from build123d import *

# Parameters (mm, degrees)
SKETCH1_R           = 16
SKETCH1_R_2         = 1.5
SKETCH1_R_3         = 5.25
SKETCH1_R_4         = 3
BOSS_EXTRUDE2_DEPTH = 3
SKETCH1_8_R         = 16
BOSS_EXTRUDE4_DEPTH = 10
SKETCH1_10_R        = 3
SKETCH1_10_R_2      = 1.5
BOSS_EXTRUDE6_DEPTH = 3
BOSS_EXTRUDE7_START = 3
SKETCH1_11_R        = 16
BOSS_EXTRUDE7_DEPTH = 57
CUT_EXTRUDE2_START  = -70
SKETCH2_R           = 1.5
CUT_EXTRUDE2_DEPTH  = 5


with BuildPart() as part:
    # Sketch1 → Boss-Extrude2 (new body)
    with BuildSketch(Plane(origin=(0, 0, 0), x_dir=(0, 0, -1), z_dir=(1, 0, 0))):
        Circle(SKETCH1_R)
        with Locations((0, 8.5)):
            Circle(SKETCH1_R_2, mode=Mode.SUBTRACT)
        with Locations((0, -8.5)):
            Circle(SKETCH1_R_2, mode=Mode.SUBTRACT)
        Circle(SKETCH1_R_3, mode=Mode.SUBTRACT)
        with Locations((8.5, 0)):
            Circle(SKETCH1_R_4, mode=Mode.SUBTRACT)
        with Locations((-8.5, 0)):
            Circle(SKETCH1_R_4, mode=Mode.SUBTRACT)
    extrude(amount=BOSS_EXTRUDE2_DEPTH)

    # Sketch1<8> → Boss-Extrude4 (add)
    with BuildSketch(Plane(origin=(0, 0, 0), x_dir=(0, 0, -1), z_dir=(1, 0, 0))):
        Circle(SKETCH1_8_R)
        with BuildLine():
            ThreePointArc((2.652911728, 9.900735294), (7.247844507, 7.247844507), (9.900735294, 2.652911728))
            ThreePointArc((9.900735294, 2.652911728), (11.069261166, 1.548837325), (11.5, 0))
            ThreePointArc((11.5, 0), (11.069261166, -1.548837325), (9.900735294, -2.652911728))
            ThreePointArc((9.900735294, -2.652911728), (7.247844507, -7.247844507), (2.652911728, -9.900735294))
            ThreePointArc((2.652911728, -9.900735294), (0, -11.5), (-2.652911728, -9.900735294))
            ThreePointArc((-2.652911728, -9.900735294), (-7.247844507, -7.247844507), (-9.900735294, -2.652911728))
            ThreePointArc((-9.900735294, -2.652911728), (-11.5, 0), (-9.900735294, 2.652911728))
            ThreePointArc((-9.900735294, 2.652911728), (-7.247844507, 7.247844507), (-2.652911728, 9.900735294))
            ThreePointArc((-2.652911728, 9.900735294), (0, 11.5), (2.652911728, 9.900735294))
        make_face(mode=Mode.SUBTRACT)
    extrude(amount=-BOSS_EXTRUDE4_DEPTH)

    # Sketch1<10> → Boss-Extrude6 (add)
    with BuildSketch(Plane(origin=(0, 0, 0), x_dir=(0, 0, -1), z_dir=(1, 0, 0))):
        with Locations((8.5, 0)):
            Circle(SKETCH1_10_R)
        with Locations((8.5, 0)):
            Circle(SKETCH1_10_R_2, mode=Mode.SUBTRACT)
        with Locations((-8.5, 0)):
            Circle(SKETCH1_10_R)
        with Locations((-8.5, 0)):
            Circle(SKETCH1_10_R_2, mode=Mode.SUBTRACT)
    extrude(amount=BOSS_EXTRUDE6_DEPTH)

    # Sketch1<11> → Boss-Extrude7 (add)
    with BuildSketch(Plane(origin=(0, 0, 0), x_dir=(0, 0, -1), z_dir=(1, 0, 0)).offset(BOSS_EXTRUDE7_START)):
        Circle(SKETCH1_11_R)
        with BuildLine():
            ThreePointArc((2.652911728, 9.900735294), (7.247844507, 7.247844507), (9.900735294, 2.652911728))
            ThreePointArc((9.900735294, 2.652911728), (11.069261166, 1.548837325), (11.5, 0))
            ThreePointArc((11.5, 0), (11.069261166, -1.548837325), (9.900735294, -2.652911728))
            ThreePointArc((9.900735294, -2.652911728), (7.247844507, -7.247844507), (2.652911728, -9.900735294))
            ThreePointArc((2.652911728, -9.900735294), (0, -11.5), (-2.652911728, -9.900735294))
            ThreePointArc((-2.652911728, -9.900735294), (-7.247844507, -7.247844507), (-9.900735294, -2.652911728))
            ThreePointArc((-9.900735294, -2.652911728), (-11.5, 0), (-9.900735294, 2.652911728))
            ThreePointArc((-9.900735294, 2.652911728), (-7.247844507, 7.247844507), (-2.652911728, 9.900735294))
            ThreePointArc((-2.652911728, 9.900735294), (0, 11.5), (2.652911728, 9.900735294))
        make_face(mode=Mode.SUBTRACT)
    extrude(amount=BOSS_EXTRUDE7_DEPTH)

    # Sketch2 → Cut-Extrude2 (cut)
    with BuildSketch(Plane.ZY.offset(10).offset(CUT_EXTRUDE2_START)):
        with Locations(Location((9.222798741, 9.222798741, 0), (0, 0, 180))):
            Circle(SKETCH2_R)
        with Locations(Location((-9.222798741, 9.222798741, 0), (0, 0, 180))):
            Circle(SKETCH2_R)
        with Locations(Location((9.222798741, -9.222798741, 0), (0, 0, 180))):
            Circle(SKETCH2_R)
        with Locations(Location((-9.222798741, -9.222798741, 0), (0, 0, 180))):
            Circle(SKETCH2_R)
    extrude(amount=CUT_EXTRUDE2_DEPTH, mode=Mode.SUBTRACT)


solid = part.part
Read the model definition and answer for the solid it produces. Units are mm, in the model's axes. A direction names the side the tool comes from. Coordinates: 2 decimals unless noted, no trailing zeros. Loops run counter-clockwise (first coordinate to the right, second up) from the corner with the lowest first, then second, coordinate; pieces in that order, holes last.
Q1. Consider probe 1 along Y at (x, z) = (42, 0); probe 2 along Y at (x, z) = (11, 1); probe 3 along Z at (x, y) = (50.5, -10). Determine where each line is inside the solid, lowest interval first.
Q2. The part is cut by section D-D on y = 8.5. Write down the section's boundary in (x, z), and give its area (3 significant figures).
Q3. Which of the six approach directions +Z, -Z, +X, -X, +Y, -Y give full straight-line access (tool end or side, diameter ignored) to faces 4 (the face through (31.1, 11.5, 0)), 5 (the face through (1.5, 1.6, -5)), 6 (the face through (-4.93, 7.195, 7.301))?
Q4. The part is cut by section A-A on x = 50.5. Write down the section's boundary in (y, z).
Q5. Each of these flat-tipped pins is pushed along its axis until it touches: pin 1 Ø0.9 at (y, z) = (9.5, 10) entering from +X; pin 2 Ø7 at (y, z) = (2, 0.5) entering from -X; pin 3 Ø5 at (x, z) = (9, 9.5) entering from -Y; pin 4 Ø2.5 at (y, z) = (-9, 8.5) entering from +X. Where does it stop, or does it pass through?
Q6. The part is cut by section B-B on z = -9. Write down the section's boundary in (x, y).
Q7. The part is cut by section C-C on y = -4. Write down the section's boundary in (x, z), and give its area (3 significant figures).
Q8. The mould has two halves that part along Y. Classify faces 1 (the face through (24.51, -15.62, 3.47)), 2 (the face through (55, 9, 9)), 3 (the face through (-10, -3, -10)): +Y half, -Y half, draft (parallel to the pull), parting line (faces both ways), or undercut.
Results below:
1. probe 1: y = -16 to -11.5, 11.5 to 16
1. probe 2: y = -15.97 to -11.33, 11.33 to 15.97
1. probe 3: z = -12.49 to -2.6, 2.6 to 12.49
2. outline: (-10, -13.56) - (60, -13.56) - (60, -10.54) - (55, -10.54) - (55, -7.91) - (60, -7.91) - (60, -5.73) - (3, -5.73) - (3, -1.5) - (0, -1.5) - (0, -5.73) - (-10, -5.73) - close; (-10, 5.73) - (0, 5.73) - (0, 1.5) - (3, 1.5) - (3, 5.73) - (60, 5.73) - (60, 7.91) - (55, 7.91) - (55, 10.54) - (60, 10.54) - (60, 13.56) - (-10, 13.56) - close
2. area: 1,090 mm2
3. face 4: +X
3. face 5: +X, -X
3. face 6: -X
4. outline: circle Ø32 at (0, 0); hole (-9.9, -2.65) arc R10.25 ccw to (-2.65, -9.9) arc R3 ccw to (2.65, -9.9) arc R10.25 ccw to (9.9, -2.65) arc R3 ccw to (9.9, 2.65) arc R10.25 ccw to (2.65, 9.9) arc R3 ccw to (-2.65, 9.9) arc R10.25 ccw to (-9.9, 2.65) arc R3 ccw to start
5. pin 1: stops at x = 55
5. pin 2: stops at x = 0
5. pin 3: stops at y = -14.39
5. pin 4: stops at x = 60
6. outline: (-10, -13.23) - (60, -13.23) - (60, -10.71) - (55, -10.71) - (55, -7.74) - (60, -7.74) - (60, -4.91) - (3, -4.91) - (3, -1.41) - (0, -1.41) - (0, -4.91) - (-10, -4.91) - close; (-10, 4.91) - (0, 4.91) - (0, 1.41) - (3, 1.41) - (3, 4.91) - (60, 4.91) - (60, 7.74) - (55, 7.74) - (55, 10.71) - (60, 10.71) - (60, 13.23) - (-10, 13.23) - close
7. outline: (-10, -15.49) - (60, -15.49) - (60, -9.44) - (3, -9.44) - (3, -3.4) - (0, -3.4) - (0, -9.44) - (-10, -9.44) - close; (-10, 9.44) - (0, 9.44) - (0, 3.4) - (3, 3.4) - (3, 9.44) - (60, 9.44) - (60, 15.49) - (-10, 15.49) - close
7. area: 884 mm2
8. face 1: parting line
8. face 2: undercut
8. face 3: draft
